```python
from build123d import *

# Parameters (mm, degrees)
REVOLVE_1_ANGLE           = 120.00000000000027
REVOLVE_2_ANGLE           = 33.00000000000007
REVOLVE_2_OTHER_WAY_ANGLE = 33.00000000000007
CUT_EXTRUDE_4_DEPTH       = 126
CUT_EXTRUDE_5_DEPTH       = 126


with BuildPart() as part:
    # Эскиз1 → Повернуть1 (revolve)
    with BuildSketch(Plane(origin=(0, 0, 0), x_dir=(0, 0, -1), z_dir=(1, 0, 0))):
        Polygon((-2e-17, 41.7), (-4.23e-15, 40.5), (89, 40.5), (89, 41.70000000000002), align=None)
    revolve(axis=Axis((0, 0, 0), (0, 0, -1)), revolution_arc=REVOLVE_1_ANGLE)

    # Эскиз3 → Повернуть2 (revolve)
    with BuildSketch(Plane(origin=(0, 0, 0), x_dir=(0, 0, 1), z_dir=(0.499999999999998, -0.8660254037844398, 0))):
        Polygon((-89, -40.5), (-215, -40.500000000000014), (-215, -41.70000000000002), (-89, -41.700000000000024), align=None)
    revolve(axis=Axis((0, 0, -89), (0, 0, 1)), revolution_arc=REVOLVE_2_ANGLE)

    # Эскиз3 → Повернуть2 other way (revolve)
    with BuildSketch(Plane(origin=(0, 0, 0), x_dir=(0, 0, 1), z_dir=(0.499999999999998, -0.8660254037844398, 0))):
        Polygon((-89, -40.5), (-215, -40.500000000000014), (-215, -41.70000000000002), (-89, -41.700000000000024), align=None)
    revolve(axis=Axis((0, 0, -89), (0, 0, -1)), revolution_arc=REVOLVE_2_OTHER_WAY_ANGLE)

    # Эскиз5 → Вырез-Вытянуть4 (cut)
    with BuildSketch(Plane(origin=(0, 0, -215), x_dir=(-1, 0, 0), z_dir=(0, 0, -1))):
        Polygon((-41.65518715609019, -1.9327138927169163), (-39.93832529078865, -1.4726821423935714), (-38.91609393559994, -3.4834404042625358), (-41.909594866084106, -3.6461306722236317), align=None)
    extrude(amount=-CUT_EXTRUDE_4_DEPTH, mode=Mode.SUBTRACT)

    # Эскиз6 → Вырез-Вытянуть5 (cut)
    with BuildSketch(Plane(origin=(0, 0, -215), x_dir=(-1, 0, 0), z_dir=(0, 0, -1))):
        Polygon((-18.830708808502447, 35.8560232843715), (-19.80637583241834, 39.49726218889504), (-16.068176634900343, 39.433464562570705), (-15.316320189263505, 34.07013113552305), align=None)
    extrude(amount=-CUT_EXTRUDE_5_DEPTH, mode=Mode.SUBTRACT)


solid = part.part
```
Geometry: final body of the model. Coordinates: model frame, mm. Round coordinates to 2 decimals unless told otherwise and drop trailing zeros. Write each loop counter-clockwise with the first axis right and the second up, starting at its lowest first coordinate (ties: lowest second). Pieces come first, ordered by that corner, then holes. Notation, with made-up numbers: M 76,9.5 L 86,9.5 A27 ccw 86,25.5 Z; hole C 73,77 d8. An arc over 180 degrees is marked long. Answer in a Markdown table with one row per item. Add a question column.
(1) Ray query, L1, parallel to X at y = 2, z = -150.5; L2, parallel to X at y = 0, z = -190; L3, parallel to Y at x = 29, z = -158. Return the intervals inside material, ascending.
(2) Contact query for flat-ended pins moving along their axis: pin 1 (5 mm diameter, centred on y = 20, z = -146, fed in from -X); pin 2 (1.8 mm diameter, centred on x = 10, y = 39, fed in from -Z); pin 3 (5 mm diameter, centred on x = 32, y = 17, fed in from +Z); pin 4 (8 mm diameter, centred on y = 12, z = -186.5, fed in from -X). Output: stop coordinate, or through.
(3) Cut plane B-B, the plane y = 19.5. Return the cut outline in (x, z), then the cut area to 3 significant figures.
(4) Cut plane A-A, the plane z = -111.5. Return the cut outline in (x, y), then the cut area to 3 significant figures.
Established:
| question | item | result |
|---|---|---|
| 1 | L1 | 40.45 to 41.65 |
| 1 | L2 | 40.5 to 41.7 |
| 1 | L3 | 28.27 to 29.96 |
| 2 | pin 1 | x = 33.67 |
| 2 | pin 2 | z = -89 |
| 2 | pin 3 | through |
| 2 | pin 4 | x = 37.21 |
| 3 | outline | M 35.5,-215 L 36.86,-215 L 36.86,0 L 35.5,0 Z |
| 3 | area | 293 mm² |
| 4 | outline | M 18.83,35.86 A40.5 cw 40.47,-1.61 L 41.66,-1.93 A41.7 ccw 19.15,37.04 Z |
| 4 | area | 55.9 mm² |
